Could you check a few things on this drawing? It's one solid part, dimensions in mm from its lowest x, y, z. A direction names the side the tool comes from. Give positions to 0.01 mm unless a question says otherwise; leave off trailing zeros. Loops run counter-clockwise (first coordinate to the right, second up) from the corner with the lowest first, then second, coordinate; pieces in that order, holes last. Notation, with made-up numbers: M -35.75,28.25 L -2.75,28.25 A21 ccw -2.75,51.25 Z; hole C -8,0 d4. An arc over 180 degrees is marked long. Answer as CSV lines item,"result". Start each with the question number.
Item 1: I want a section at A-A on y = 10. List the corners of the cut face in (x, z) for me, plus the area to 4 significant figures.
Item 2: I want a section at D-D on z = 29. List the corners of the cut face in (x, y) for me, plus the area to 3 significant figures.
Item 3: Will these pins go through, and if not, where does the flat tip stop? P1, Ø1, axis at y = 3, z = 4, coming from the -X side; P2, Ø3, axis at x = 30, y = 2, coming from the +Z side; P3, Ø3.5, axis at x = 2.5, y = 5, coming from the -Z side; P4, Ø2, axis at x = 2, y = 2, coming from the +Z side.
Item 4: For the marked faces 1, 2, 3 and 4, which set-ups out of +Z, -Z, +X, -X, +Y, -Y let a thin tool reach every point of the face, with its end or its side?
Item 5: I want a section at B-B on x = 2. List the corners of the cut face in (y, z) for me, plus the area to 3 significant figures.
Item 6: I want a section at C-C on x = 21.79. List the corners of the cut face in (y, z) for me.
Item 7: If I drill on line 1 along Y through (x, z) = (30, 21); line 2 along X through (y, z) = (10, 20.95); line 3 along Z through (x, y) = (19.5, 3.5), over which ranges is the centre line in solid material (lowest first)? Write a range as from..to.
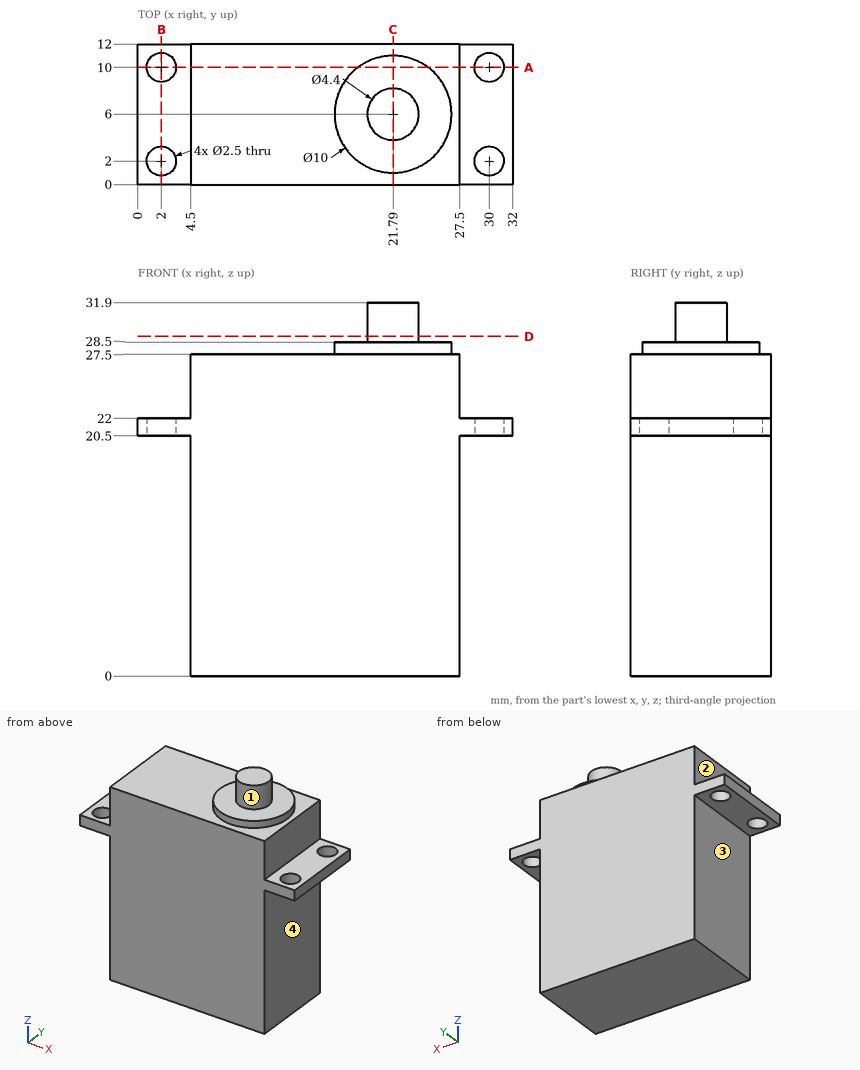
Result:
1,outline,"M 0,20.5 L 0.75,20.5 L 0.75,22 L 0,22 Z; M 3.25,20.5 L 4.5,20.5 L 4.5,0 L 27.5,0 L 27.5,20.5 L 28.75,20.5 L 28.75,22 L 27.5,22 L 27.5,27.5 L 24.79,27.5 L 24.79,28.5 L 18.79,28.5 L 18.79,27.5 L 4.5,27.5 L 4.5,22 L 3.25,22 Z; M 31.25,20.5 L 32,20.5 L 32,22 L 31.25,22 Z"
1,area,"644.5 mm^2"
2,outline,"C 21.79,6 d4.4"
2,area,"15.2 mm^2"
3,P1,"x = 4.5"
3,P2,"z = 22"
3,P3,"z = 20.5"
3,P4,"through"
4,face 1,"+Z"
4,face 2,"+Z, -X, +Y, -Y"
4,face 3,"-Z, -X, +Y, -Y"
4,face 4,"-Z, +X, +Y, -Y"
5,outline,"M 0,20.5 L 0.75,20.5 L 0.75,22 L 0,22 Z; M 3.25,20.5 L 8.75,20.5 L 8.75,22 L 3.25,22 Z; M 11.25,20.5 L 12,20.5 L 12,22 L 11.25,22 Z"
5,area,"10.5 mm^2"
6,outline,"M 0,0 L 12,0 L 12,27.5 L 11,27.5 L 11,28.5 L 8.2,28.5 L 8.2,31.9 L 3.8,31.9 L 3.8,28.5 L 1,28.5 L 1,27.5 L 0,27.5 Z"
7,line 1,"0..0.75, 3.25..8.75, 11.25..12"
7,line 2,"0..0.75, 3.25..28.75, 31.25..32"
7,line 3,"0..28.5"
